from build123d import *

# Parameters (mm, degrees)
SKETCH1_R           = 4
BOSS_EXTRUDE1_DEPTH = 12.5
CUT_EXTRUDE1_REACH  = 85.156
SKETCH4_W           = 25.5
SKETCH4_H           = 5
SKETCH5_R           = 4
CUT_EXTRUDE2_DEPTH  = 80.522425


with BuildPart() as part:
    # Sketch1 → Boss-Extrude1 (new, symmetric)
    # profile 1 of 3: a face of its own
    with BuildSketch(Plane(origin=(0, 0, 0), x_dir=(1, 0, 0), z_dir=(0, 1, 0))):
        Circle(SKETCH1_R)
    # profile 2 of 3: a face of its own
    with BuildSketch(Plane(origin=(0, 0, 0), x_dir=(1, 0, 0), z_dir=(0, 1, 0))):
        with BuildLine():
            Line((-34.72, 8), (0, 8))
            ThreePointArc((0, 8), (8, 0), (0, -8))
            Line((0, -8), (-34.72, -8))
            ThreePointArc((-34.72, -8), (-42.72, 0), (-34.72, 8))
        make_face()
        with Locations(Location((-34.72, 0, 0), (0, 0, 270))):
            Circle(SKETCH1_R, mode=Mode.SUBTRACT)
    # profile 3 of 3: a face of its own
    with BuildSketch(Plane(origin=(0, 0, 0), x_dir=(1, 0, 0), z_dir=(0, 1, 0))):
        with BuildLine():
            Line((-7.465452, 2.875245), (13.424548, 57.115245))
            ThreePointArc((13.424548, 57.115245), (23.765245, 61.705452), (28.355452, 51.364755))
            Line((28.355452, 51.364755), (7.465452, -2.875245))
            ThreePointArc((7.465452, -2.875245), (-2.875245, -7.465452), (-7.465452, 2.875245))
        make_face()
        with Locations(Location((20.89, 54.24, 0), (0, 0, 270))):
            Circle(SKETCH1_R, mode=Mode.SUBTRACT)
    extrude(amount=BOSS_EXTRUDE1_DEPTH, both=True)

    # Sketch4 → Cut-Extrude1 (cut, up to next)
    with BuildSketch(Plane.XY.offset(8), mode=Mode.PRIVATE) as cut_extrude1_sk1:
        with Locations((-29.97, 0)):
            Rectangle(SKETCH4_W, SKETCH4_H)
    cut_extrude1_tool1 = extrude(cut_extrude1_sk1.sketch, amount=-CUT_EXTRUDE1_REACH, mode=Mode.PRIVATE) & part.part
    add(cut_extrude1_tool1.solids().sort_by_distance((-29.97, 0, 8))[0], mode=Mode.SUBTRACT)

    # Sketch5 → Cut-Extrude2 (cut, through all)
    with BuildSketch(Plane(origin=(0, 12.5, 0), x_dir=(1, 0, 0), z_dir=(0, 1, 0))):
        with Locations(Location((0, 0, 0), (0, 0, 270))):
            Circle(SKETCH5_R)
    extrude(amount=-CUT_EXTRUDE2_DEPTH, mode=Mode.SUBTRACT)


solid = part.part
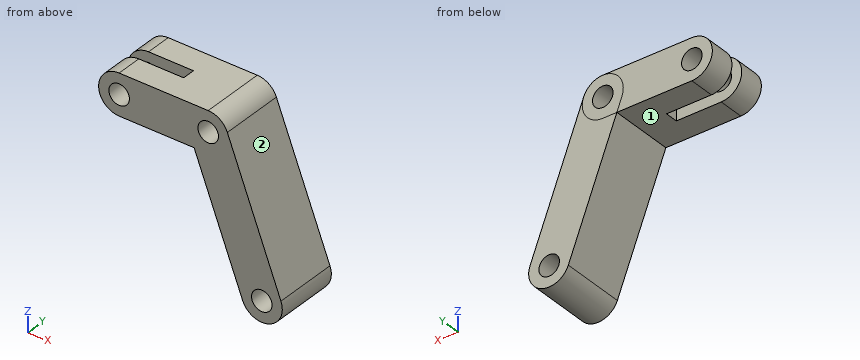
Input: part model. Units: mm. Frame: model coordinates. Face numbers are marked on the shaded views. A direction names the side the tool comes from. Coordinates: 2 decimals unless noted, no trailing zeros. Loops run counter-clockwise (first coordinate to the right, second up) from the corner with the lowest first, then second, coordinate; pieces in that order, holes last.
Q1. Contact query for flat-ended pins moving along their axis: pin 1 (1.5 mm diameter, centred on y = -0.5, z = -1, fed in from -X); pin 2 (7.5 mm diameter, centred on x = -14.5, y = -4, fed in from -Z); pin 3 (5 mm diameter, centred on y = 4.5, z = -38, fed in from +X). Output: stop coordinate, or through.
Q2. Cut plane A-A (y = 8). Output: boundary loops of the cut face in (x, z), then the cut area to 3 significant figures.
Q3. Material intervals for line 1 (Y direction, x = -17.5, z = 1); line 2 (X direction, y = 10.5, z = 1); line 3 (X direction, y = 0, z = 1), sorted ascending.
Q4. Cut plane B-B (z = 0). Output: boundary loops of the cut face in (x, y).
Q5. Cut plane C-C (x = 1). Output: boundary loops of the cut face in (y, z), then the cut area to 3 significant figures.
Q6. Set-up query: the marked faces 1 and 2. Return all of +Z, -Z, +X, -X, +Y, -Y with unobstructed straight access to the full face (end or side cutting, diameter ignored); none if empty.
Q7. Cut plane D-D (z = -54.24). Output: boundary loops of the cut face in (x, y).
Working result:
1. pin 1: stops at x = -17.22
1. pin 2: stops at z = -8
1. pin 3: stops at x = 24.17
2. outline: (-34.72, -8) - (-5.49, -8) - (13.42, -57.12) arc R8 ccw to (28.36, -51.36) - (7.47, 2.88) arc R8 ccw to (0, 8) - (-34.72, 8) arc R8 ccw to start; hole circle Ø8 at (-34.72, 0); hole circle Ø8 at (0, 0); hole circle Ø8 at (20.89, -54.24)
2. area: 1,530 mm2
3. line 1: y = -12.5 to -2.5, 2.5 to 12.5
3. line 2: x = -42.66 to -38.59, -30.85 to -3.87, 3.87 to 8.19
3. line 3: x = -17.22 to -3.87, 3.87 to 8.19
4. outline: (-42.72, -12.5) - (-38.72, -12.5) - (-38.72, -2.5) - (-42.72, -2.5) - close; (-42.72, 2.5) - (-38.72, 2.5) - (-38.72, 12.5) - (-42.72, 12.5) - close; (-30.72, -12.5) - (-4, -12.5) - (-4, 12.5) - (-30.72, 12.5) - (-30.72, 2.5) - (-17.22, 2.5) - (-17.22, -2.5) - (-30.72, -2.5) - close; (4, -12.5) - (8.57, -12.5) - (8.57, 12.5) - (4, 12.5) - close
5. outline: (-12.5, -24.86) - (12.5, -24.86) - (12.5, -3.87) - (-12.5, -3.87) - close; (-12.5, 3.87) - (12.5, 3.87) - (12.5, 7.94) - (-12.5, 7.94) - close
5. area: 626 mm2
6. face 1: -Z, -X, +Y, -Y
6. face 2: +Z, +X, +Y, -Y
7. outline: (12.32, -12.5) - (16.89, -12.5) - (16.89, 12.5) - (12.32, 12.5) - close; (24.89, -12.5) - (28.89, -12.5) - (28.89, 12.5) - (24.89, 12.5) - close
